```python
from build123d import *

# Parameters (mm, degrees)
SALIENTE_EXTRUIR2_DEPTH = 200
VACIADO2_T              = -3
CROQUIS6_R              = 8.2
CORTAR_EXTRUIR4_DEPTH   = 80
CROQUIS2_R              = 8.02
CORTAR_EXTRUIR5_DEPTH   = 3
CORTAR_EXTRUIR6_START   = -3
CROQUIS5_R              = 8.02
CORTAR_EXTRUIR6_DEPTH   = 3
CROQUIS7_W              = 7.4
CROQUIS7_H              = 7.4
CORTAR_EXTRUIR11_DEPTH  = 3
CROQUIS8_W              = 7.04
CROQUIS8_H              = 7.04
CORTAR_EXTRUIR12_DEPTH  = 3
CROQUIS9_W              = 35
CROQUIS9_H              = 35
CORTAR_EXTRUIR13_DEPTH  = 3
CROQUIS15_W             = 6
CROQUIS15_H             = 3
SALIENTE_EXTRUIR3_DEPTH = 75


with BuildPart() as part:
    # Croquis1 → Saliente-Extruir2 (new body)
    with BuildSketch(Plane(origin=(0, 0, 0), x_dir=(1, 0, 0), z_dir=(0, 1, 0))):
        Polygon((0, 0), (200, 0), (200, 80), (160, 80), align=None)
    extrude(amount=SALIENTE_EXTRUIR2_DEPTH)

    # Vaciado2
    vaciado2_openings = [part.faces().sort_by_distance(p)[0] for p in [
        (200, 100, -40),
    ]]
    offset(amount=VACIADO2_T, openings=vaciado2_openings, kind=Kind.INTERSECTION)

    # Croquis6 → Cortar-Extruir4 (cut)
    with BuildSketch(Plane(origin=(0, 0, 0), x_dir=(0, 0, -1), z_dir=(1, 0, 0))):
        with Locations(Location((30, 88.575, 0), (0, 0, 180))):
            Circle(CROQUIS6_R)
        with Locations(Location((30, 111.425, 0), (0, 0, 180))):
            Circle(CROQUIS6_R)
    extrude(amount=CORTAR_EXTRUIR4_DEPTH, mode=Mode.SUBTRACT)

    # Croquis2 → Cortar-Extruir5 (cut)
    with BuildSketch(Plane(origin=(0, 200, 0), x_dir=(1, 0, 0), z_dir=(0, 1, 0))):
        with Locations(Location((88.011571484, 15, 0), (0, 0, 270))):
            Circle(CROQUIS2_R)
        with Locations(Location((115.531571484, 15, 0), (0, 0, 270))):
            Circle(CROQUIS2_R)
    extrude(amount=-CORTAR_EXTRUIR5_DEPTH, mode=Mode.SUBTRACT)

    # Croquis5 → Cortar-Extruir6 (cut)
    with BuildSketch(Plane.XZ.offset(CORTAR_EXTRUIR6_START)):
        with Locations(Location((88.011571484, -15, 0), (0, 0, 90))):
            Circle(CROQUIS5_R)
        with Locations(Location((115.531571484, -15, 0), (0, 0, 90))):
            Circle(CROQUIS5_R)
    extrude(amount=CORTAR_EXTRUIR6_DEPTH, mode=Mode.SUBTRACT)

    # Croquis7 → Cortar-Extruir11 (cut)
    with BuildSketch(Plane.XY):
        with Locations((18.7, 13.7)):
            Rectangle(CROQUIS7_W, CROQUIS7_H)
    cortar_extruir11 = extrude(amount=-CORTAR_EXTRUIR11_DEPTH, mode=Mode.SUBTRACT)

    # Simetría5: Cortar-Extruir11 across plane
    add(cortar_extruir11.mirror(Plane.ZX.offset(100)), mode=Mode.SUBTRACT)

    # Croquis8 → Cortar-Extruir12 (cut)
    with BuildSketch(Plane.XY):
        with Locations((18.52, 100)):
            Rectangle(CROQUIS8_W, CROQUIS8_H)
    extrude(amount=-CORTAR_EXTRUIR12_DEPTH, mode=Mode.SUBTRACT)

    # Croquis9 → Cortar-Extruir13 (cut)
    with BuildSketch(Plane.XY):
        with Locations((174.5, 174.5)):
            Rectangle(CROQUIS9_W, CROQUIS9_H)
    cortar_extruir13 = extrude(amount=-CORTAR_EXTRUIR13_DEPTH, mode=Mode.SUBTRACT)

    # Simetría6: Cortar-Extruir13 across plane
    add(cortar_extruir13.mirror(Plane.ZX.offset(100)), mode=Mode.SUBTRACT)

    # Croquis15 → Saliente-Extruir3 (add)
    with BuildSketch(Plane(origin=(0, 0, -3), x_dir=(-1, 0, 0), z_dir=(0, 0, -1))):
        with Locations((-197, 4.5)):
            Rectangle(CROQUIS15_W, CROQUIS15_H)
    saliente_extruir3 = extrude(amount=SALIENTE_EXTRUIR3_DEPTH)

    # Simetría7: Saliente-Extruir3 across plane
    add(saliente_extruir3.mirror(Plane.ZX.offset(100)))

    # Croquis18 → Refrentado para tornillo tapón con cabeza plana de clavija de M33 (revolve, cut)
    with BuildSketch(Plane(origin=(196, 4, 0), x_dir=(0, -1, 0), z_dir=(1, 0, 0))):
        Polygon((0, 0), (0, 11.021463052), (1.7, 10), (1.7, 1.66), (3.36, 0), align=None)
    refrentado_para_tornillo_tap_n_con_cabez = revolve(axis=Axis((196, 4, 6.35), (0, 0, -1)), mode=Mode.SUBTRACT)

    # Simetría8: Refrentado para tornillo tapón con cabeza plana de clavija de M33 across plane
    add(refrentado_para_tornillo_tap_n_con_cabez.mirror(Plane.ZX.offset(100)), mode=Mode.SUBTRACT)

    # Simetría9: Refrentado para tornillo tapón con cabeza plana de clavija de M33 across plane
    add(refrentado_para_tornillo_tap_n_con_cabez.mirror(Plane(origin=(100, 0, 0), x_dir=(0, 0, 1), z_dir=(1, 0, 0))), mode=Mode.SUBTRACT)

    # Simetría9 copy 1 sketch → Simetría9 copy 1 (revolve, cut)
    with BuildSketch(Plane(origin=(4, 196, 0), x_dir=(0, 1, 0), z_dir=(-1, 0, 0))):
        Polygon((0, 0), (0, 11.021463052), (1.7, 10), (1.7, 1.66), (3.36, 0), align=None)
    revolve(axis=Axis((4, 196, 6.35), (0, 0, -1)), mode=Mode.SUBTRACT)


solid = part.part
```
Source: CAD feature listing. Evaluate the final solid. Frame: model axes, mm. A direction names the side the tool comes from. Give positions to 0.01 mm unless a question says otherwise; leave off trailing zeros. Loops run counter-clockwise (first coordinate to the right, second up) from the corner with the lowest first, then second, coordinate; pieces in that order, holes last. Notation, with made-up numbers: (87.25, -3) - (115.25, -3) arc R16 ccw to (115.25, 18) - close; hole circle Ø7 at (66, 36). An arc over 180 degrees is marked (long way). Use CSV: the item, a comma, the result in double quotes. Start each with the question number.
1. Section C-C (y = 135). Output: boundary loops of the cut face in (x, z), then the cut area to 3 significant figures.
2. Pin query (flat end, axial travel): pin 1 (1.5 mm diameter, centred on y = 101, z = -2, fed in from -X); pin 2 (5.5 mm diameter, centred on x = 4, y = 4, fed in from +Z); pin 3 (0.5 mm diameter, centred on y = 90, z = -37.5, fed in from -X). Return the tip coordinate at first contact, or that it passes through.
3. Ray query, L1, parallel to Y at x = 196, z = -6.5; L2, parallel to Y at x = 109.5, z = -28; L3, parallel to X at y = 4, z = -2. Return the intervals inside material, ascending.
4. Section A-A (y = 185). Output: boundary loops of the cut face in (x, z).
5. Section D-D (x = 85.5). Output: boundary loops of the cut face in (y, z), then the cut area to 3 significant figures.
6. Section B-B (z = -15). Output: boundary loops of the cut face in (x, y).
7. Draft query along Z for faces 4 (the cylindrical face through (61.715, 103.247, -29.403)), 5 (the conical face through (5.971, 195.741, -1.372)), 6 (the flat face through (81.12, 98.6, -40.56)), 7 (the flat face through (87.744, 98.642, -40.518)). Return one class per face: +Z half, -Z half, draft (parallel to the pull), parting line (faces both ways), or undercut.
8. Reachability of faces 1 (the cylindrical face through (84.94, 198.52, -7.59)), 2 (the cylindrical face through (61.715, 80.397, -29.403)), 3 (the flat face through (142, 197, -32)) from +Z, -Z, +X, -X, +Y, -Y: full face, straight path, thin tool, end or side. Return the list, or none.
Response:
1,outline,"(0, 0) - (160, -80) - (200, -80) - (200, -77) - (160.71, -77) - (12.71, -3) - (200, -3) - (200, 0) - close"
1,area,"1,220 mm²"
2,pin 1,"x = 2.5"
2,pin 2,"z = -0.61"
2,pin 3,"x = 80"
3,L1,"0 to 2.3, 5.7 to 6, 194 to 194.3, 197.7 to 200"
3,L2,"0 to 3, 197 to 200"
3,L3,"5.7 to 194.3, 197.7 to 200"
4,outline,"(0, 0) - (160, -80) - (200, -80) - (200, -77) - (160.71, -77) - (12.71, -3) - (15, -3) - (15, 0) - close; (22.4, -3) - (157, -3) - (157, 0) - (22.4, 0) - close; (192, -3) - (200, -3) - (200, 0) - (192, 0) - close"
5,outline,"(0, -42.75) - (200, -42.75) - (200, -22.62) - (197, -22.62) - (197, -39.4) - (3, -39.4) - (3, -22.62) - (0, -22.62) - close; (0, -7.38) - (3, -7.38) - (3, -3) - (197, -3) - (197, -7.38) - (200, -7.38) - (200, 0) - (0, 0) - close"
5,area,"1,400 mm²"
6,outline,"(30, 0) - (79.99, 0) - (79.99, 3) - (36.71, 3) - (36.71, 197) - (79.99, 197) - (79.99, 200) - (30, 200) - close; (96.03, 0) - (107.51, 0) - (107.51, 3) - (96.03, 3) - close; (96.03, 197) - (107.51, 197) - (107.51, 200) - (96.03, 200) - close; (123.55, 0) - (200, 0) - (200, 6) - (194, 6) - (194, 3) - (123.55, 3) - close; (123.55, 197) - (194, 197) - (194, 194) - (200, 194) - (200, 200) - (123.55, 200) - close"
7,face 4,"undercut"
7,face 5,"+Z half"
7,face 6,"-Z half"
7,face 7,"undercut"
8,face 1,"+Y, -Y"
8,face 2,"-X"
8,face 3,"none"
